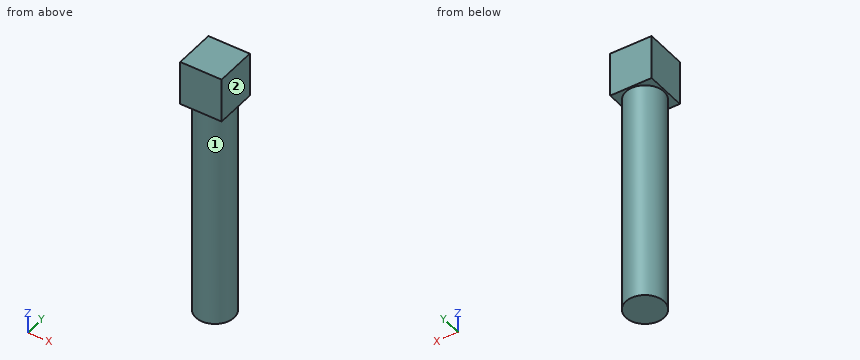
```python
from build123d import *

# Parameters (mm, degrees)
SKETCH1_R           = 6
BOSS_EXTRUDE1_DEPTH = 70
SKETCH2_W           = 13
SKETCH2_H           = 13
BOSS_EXTRUDE2_DEPTH = 14


with BuildPart() as part:
    # Sketch1 → Boss-Extrude1 (new body)
    with BuildSketch(Plane.XY):
        Circle(SKETCH1_R)
    extrude(amount=BOSS_EXTRUDE1_DEPTH)

    # Sketch2 → Boss-Extrude2 (add)
    with BuildSketch(Plane.XY.offset(84)):
        Rectangle(SKETCH2_W, SKETCH2_H)
    extrude(amount=-BOSS_EXTRUDE2_DEPTH)


solid = part.part
```
The model under review builds one solid part; all positions refer to its coordinate system, in mm. Face numbers are marked on the shaded views. A direction names the side the tool comes from. Round coordinates to 2 decimals unless told otherwise and drop trailing zeros. Loops run counter-clockwise (first coordinate to the right, second up) from the corner with the lowest first, then second, coordinate; pieces in that order, holes last. Notation, with made-up numbers: (41, 69) -> (96, 69) arc R29 ccw to (96, 103) -> close; hole circle Ø5 at (73, 66). An arc over 180 degrees is marked (long way). Answer as a JSON object with one key per item and string values. Group by question number.
1) For pin 1 Ø6 at (y, z) = (3, 45.5) entering from -X; pin 2 Ø1 at (x, z) = (-3.5, 13) entering from -Y; pin 3 Ø1 at (y, z) = (-1.5, 25.5) entering from +X, all flat-tipped, find the tip position at first contact; note any pin that passes through.
2) For line 1 (Z direction, x = -4.25, y = -4.5); line 2 (Y direction, x = 0, z = 39); line 3 (X direction, y = -0.25, z = 15.5), list the stretches that pass through material, from the lowest coordinate up. Write a range as [from, to].
3) For the marked faces 1 and 2, list the 3-axis set-ups (+Z, -Z, +X, -X, +Y, -Y) from which the entire face can be reached by the end or side of a thin tool; tool diameter is ignored.
4) We need section C-C on z = 48. Write out the cut boundary in (x, y).
5) We need section A-A on y = 0. Write out the cut boundary in (x, z).
Result set:
{
 "1": {"pin 1": "x = -6", "pin 2": "y = -5.2", "pin 3": "x = 5.92"},
 "2": {"line 1": "[70, 84]", "line 2": "[-6, 6]", "line 3": "[-5.99, 5.99]"},
 "3": {"face 1": "-Z", "face 2": "+Z, -Z, +X, +Y, -Y"},
 "4": {"outline": "circle Ø12 at (0, 0)"},
 "5": {"outline": "(-6.5, 70) -> (-6, 70) -> (-6, 0) -> (6, 0) -> (6, 70) -> (6.5, 70) -> (6.5, 84) -> (-6.5, 84) -> close"}
}
